For this review, take the finished solid that the model builds, in its own axes (mm). Face numbers are marked on the shaded views. A direction names the side the tool comes from. Give positions to 0.01 mm unless a question says otherwise; leave off trailing zeros. Order: outer loops, then holes, each group sorted by start corner. A loop starts at its lowest first (then second) coordinate and runs counter-clockwise, first axis right, second up.
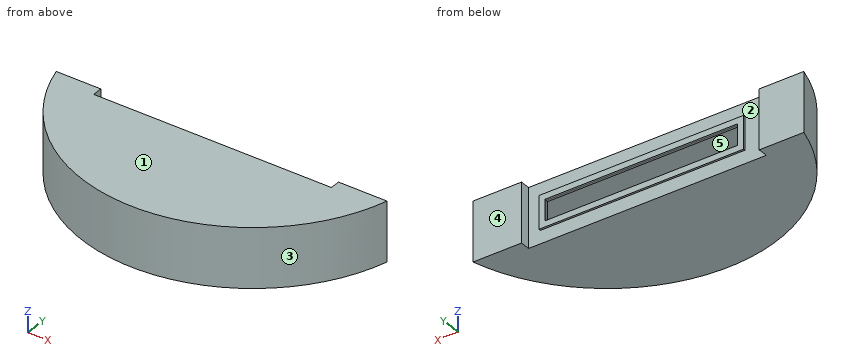
from build123d import *

# Parameters (mm, degrees)
PAD002_DEPTH   = 30
SKETCH002_W    = 119.834198
SKETCH002_H    = 56.27994
POCKET_DEPTH   = 5
SKETCH003_W    = 103.127247
SKETCH003_H    = 16.613194
PAD003_DEPTH   = 1
THICKNESS001_T = -3


with BuildPart() as part:
    # Sketch001 → Pad002 (new body)
    with BuildSketch(Plane.XY):
        with BuildLine():
            ThreePointArc((-68.184374, 10.831253), (15.204238, -53.178213), (98.592851, 10.831253))
            Line((-68.184374, 10.831253), (98.592851, 10.831253))
        make_face()
    extrude(amount=PAD002_DEPTH)

    # Sketch002 (on Face2 of Pad002) → Pocket (cut)
    with BuildSketch(Plane(origin=(0, 10.831253, 0), x_dir=(-1, 0, 0), z_dir=(0, 1, 0))):
        with Locations((-14.19677, 16.75429)):
            Rectangle(SKETCH002_W, SKETCH002_H)
    extrude(amount=-POCKET_DEPTH, mode=Mode.SUBTRACT)

    # Sketch003 (on Face8 of Pocket) → Pad003 (join)
    with BuildSketch(Plane(origin=(0, 5.831253, 0), x_dir=(-1, 0, 0), z_dir=(0, 1, 0))):
        with Locations((-16.664015, 14.938789)):
            Rectangle(SKETCH003_W, SKETCH003_H)
    extrude(amount=PAD003_DEPTH)

    # Thickness001
    thickness001_openings = [part.faces().sort_by_distance(p)[0] for p in [
        (16.664015, 6.831253, 14.938789),
    ]]
    offset(amount=THICKNESS001_T, openings=thickness001_openings)


solid = part.part
1) We need section A-A on y = -48. Give the boundary of the cut face in (x, z).
Answer sheet:
outline: (-14.24, 0) - (44.65, 0) - (44.65, 30) - (-14.24, 30) - close; hole (-3.72, 3) - (34.13, 3) - (34.13, 27) - (-3.72, 27) - close
2) Draft analysis for pull direction X (two halves, no side actions). For the marked faces 1, 2 and 3, state which applies: +X half, -X half, draft (parallel to the pull), parting line (faces both ways), or undercut.
Answer sheet:
face 1: draft
face 2: undercut
face 3: parting line
3) Clearance check with flat-ended pins moving along their axes: pin 1 (1.1 mm diameter, centred on y = 6.5, z = 12.5, fed in from +X); pin 2 (5 mm diameter, centred on y = -44, z = 9, fed in from +X); pin 3 (1.5 mm diameter, centred on x = -38.5, z = 4, fed in from -Y). State where each tip first meets the part, or that it passes through.
Answer sheet:
pin 1: stops at x = 97.49
pin 2: stops at x = 58.56
pin 3: stops at y = -35.03
4) We need section B-B on z = 14.5. Give the boundary of the cut face in (x, y).
Answer sheet:
outline: (-68.18, 10.83) arc R86.32 ccw to (98.59, 10.83) - (74.11, 10.83) - (74.11, 5.83) - (68.23, 5.83) - (68.23, 6.83) - (65.23, 6.83) - (65.23, 5.83) arc R3 ccw to (68.23, 2.83) - (74.11, 2.83) arc R3 ccw to (77.11, 5.83) - (77.11, 7.83) - (94.59, 7.83) arc R83.32 cw to (-64.18, 7.83) - (-48.72, 7.83) - (-48.72, 5.83) arc R3 ccw to (-45.72, 2.83) - (-34.9, 2.83) arc R3 ccw to (-31.9, 5.83) - (-31.9, 6.83) - (-34.9, 6.83) - (-34.9, 5.83) - (-45.72, 5.83) - (-45.72, 10.83) - close
5) We need section C-C on x = -43. Give the boundary of the cut face in (y, z).
Answer sheet:
outline: (-30.6, 0) - (5.83, 0) - (5.83, 30) - (-30.6, 30) - close; hole (-26.48, 3) - (2.83, 3) - (2.83, 27) - (-26.48, 27) - close
6) To check wall thickness, follow line 1 (Z direction, x = 20.5, y = -30); line 2 (Y direction, x = -61, z = 7.5); line 3 (X direction, y = -1, z = 11.75). State the ranges of each line that lie inside material, in increasing order.
Answer sheet:
line 1: z = 0 to 3, 27 to 30
line 2: y = -7.41 to -0.55, 7.83 to 10.83
line 3: x = -64.08 to -60.8, 91.21 to 94.49
7) We need section D-D on x = 37. Give the boundary of the cut face in (y, z), then the cut area to 3 significant figures.
Answer sheet:
outline: (-50.38, 0) - (5.83, 0) - (5.83, 6.63) - (6.83, 6.63) - (6.83, 9.63) - (5.83, 9.63) arc R3 ccw to (2.83, 6.63) - (2.83, 3) - (-47.28, 3) - (-47.28, 27) - (2.83, 27) - (2.83, 23.25) arc R3 ccw to (5.83, 20.25) - (6.83, 20.25) - (6.83, 23.25) - (5.83, 23.25) - (5.83, 30) - (-50.38, 30) - close
area: 454 mm2
8) Tool access review of the marked faces 4 and 5: name each direction out of +Z, -Z, +X, -X, +Y, -Y from which nothing blocks a thin tool from reaching the whole face with its end or side.
Answer sheet:
face 4: +Z, -Z, +X, -X, +Y
face 5: none
